Here's how the part is built. I have some questions about the finished solid (model axes, mm). A direction names the side the tool comes from. Round coordinates to 2 decimals unless told otherwise and drop trailing zeros. Order: outer loops, then holes, each group sorted by start corner. A loop starts at its lowest first (then second) coordinate and runs counter-clockwise, first axis right, second up. Notation, with made-up numbers: M -7.75,13 L 8.25,13 A9 cw 8.25,20 Z; hole C 27.25,4.25 d6. An arc over 180 degrees is marked long. Answer as CSV lines item,"result". Start each with the question number.
```python
from build123d import *

# Parameters (mm, degrees)
F1_DEPTH  = 6.096
F2_R      = 4.7625
F3_DEPTH  = 140.971
F4_R      = 3.175
F5_DEPTH  = 117.476
F6_R      = 2.0193
F6_R_2    = 1.6002
F7_DEPTH  = 12.7
F8_R      = 1.6002
F8_R_2    = 2.0193
F9_DEPTH  = 10.16
F10_R     = 1.6002
F10_R_2   = 2.0193
F11_DEPTH = 10.16


with BuildPart() as f1:
    # F0 (on Front) → F1 (new body, symmetric)
    with BuildSketch(Plane.XZ):
        with BuildLine():
            Line((-70.485, 0), (0, 0))
            Line((0, 0), (70.485, 0))
            Line((70.485, 0), (70.485, 117.475))
            Line((70.485, 117.475), (57.785, 117.475))
            Line((57.785, 117.475), (57.785, 45.3136))
            ThreePointArc((57.785, 45.3136), (57.4966846366, 43.4219130898), (56.6579198847, 41.7020064627))
            Line((56.6579198847, 41.7020064627), (38.4969198847, 15.4384064627))
            ThreePointArc((38.4969198847, 15.4384064627), (36.2226336699, 13.426117046), (33.274, 12.7))
            Line((33.274, 12.7), (0, 12.7))
            Line((0, 12.7), (-33.274, 12.7))
            ThreePointArc((-33.274, 12.7), (-36.2226336699, 13.426117046), (-38.4969198847, 15.4384064627))
            Line((-38.4969198847, 15.4384064627), (-56.6579198847, 41.7020064627))
            ThreePointArc((-56.6579198847, 41.7020064627), (-57.4966846366, 43.4219130898), (-57.785, 45.3136))
            Line((-57.785, 45.3136), (-57.785, 117.475))
            Line((-57.785, 117.475), (-70.485, 117.475))
            Line((-70.485, 117.475), (-70.485, 0))
        make_face()
    extrude(amount=F1_DEPTH, both=True)

    # F2 (on face) → F3 (cut, through all)
    with BuildSketch(Plane.YZ.offset(70.485)):
        with Locations((0, 111.125)):
            Circle(F2_R)
        with Locations((0, 85.725)):
            Circle(F2_R)
    extrude(amount=-F3_DEPTH, mode=Mode.SUBTRACT)

    # F4 (on face) → F5 (cut, through all)
    with BuildSketch(Plane(origin=(0, 0, 0), x_dir=(1, 0, 0), z_dir=(0, 0, -1))):
        with Locations((-22.225, 0)):
            Circle(F4_R)
        with Locations((22.225, 0)):
            Circle(F4_R)
    extrude(amount=-F5_DEPTH, mode=Mode.SUBTRACT)

    # F6 (on face) → F7 (cut)
    with BuildSketch(Plane(origin=(0, 0, 0), x_dir=(1, 0, 0), z_dir=(0, 0, -1))):
        with Locations((-50.8, 0)):
            Circle(F6_R)
        with Locations((-58.293, 0)):
            Circle(F6_R_2)
        with Locations((50.8, 0)):
            Circle(F6_R)
        with Locations((58.293, 0)):
            Circle(F6_R_2)
    extrude(amount=-F7_DEPTH, mode=Mode.SUBTRACT)

    # F8 (on face) → F9 (cut)
    with BuildSketch(Plane.YZ.offset(70.485)):
        with Locations((0, 6.35)):
            Circle(F8_R)
        with Locations((0, 47.625)):
            Circle(F8_R)
        with Locations((0, 15.875)):
            Circle(F8_R_2)
    extrude(amount=-F9_DEPTH, mode=Mode.SUBTRACT)

    # F10 (on face) → F11 (cut)
    with BuildSketch(Plane(origin=(-70.485, 0, 0), x_dir=(0, -1, 0), z_dir=(-1, 0, 0))):
        with Locations((0, 6.35)):
            Circle(F10_R)
        with Locations((0, 15.875)):
            Circle(F10_R_2)
        with Locations((0, 47.625)):
            Circle(F10_R)
    extrude(amount=-F11_DEPTH, mode=Mode.SUBTRACT)


solid = f1.part
```
Item 1: If we section it at D-D on y = 0: Count the separate pieces of the cut face and the enclosed holes in it, and give its area (3 significant figures).
Item 2: If we section it at A-A on z = 92: Please give me the cut outline in (x, y) (3 decimals), and give its area (3 significant figures).
Item 3: Which directions (+Z, -Z, +X, -X, +Y, -Y) give clear straight access to the entire face, cutting with the end or side of a thin tool? Please do faces 4 (the cylindrical face through (-65.476, 0.438, 13.904)), 5 (the flat face through (0, 0, 12.7)), 6 (the cylindrical face through (65.48, -0.35, 4.79)).
Item 4: If we section it at B-B on z = 6.35: Please give me the cut outline in (x, y) (3 decimals), and give its area (3 significant figures).
Item 5: For P1, Ø1.9, axis at y = 0, z = 47.625, coming from the +X side (3 decimals); P2, Ø4, axis at x = 58.293, y = 0, coming from the -Z side; P3, Ø3, axis at x = 45.5, y = 2.5, coming from the +Z side; P4, Ø1.6, axis at y = 0, z = 6.5, coming from the -X side (3 decimals), each with a flat end and sliding along its axis, tell me the tip position at first contact or that it passes through.
Item 6: If I drill on line 1 along Z through (x, y) = (67.25, 0) (1 decimal); line 2 along Z through (x, y) = (-59.5, 0.25) (3 decimals); line 3 along X through (y, z) = (5, 105) (3 decimals), over which ranges is the centre line in solid material (lowest first)?
Item 7: If we section it at C-C on x = -22.5: Please give me the cut outline in (y, z).
Item 8: We'd pull the mould along Y, two halves only. Please class faces 1 (the flat face through (47.7, -0.09, 28.75)), 2 (the flat face through (-6, -6.096, 11)), 3 (the cylindrical face through (-65.48, 0.35, 4.79)): pulls with the +Y half, pulls with the -Y half, needs draft (parallel to the pull), parting line crosses it, or undercut.
Geometry says:
1,separate pieces,"7"
1,enclosed holes,"0"
1,area,"4,060 mm²"
2,outline,"M -70.485,-6.096 L -57.785,-6.096 L -57.785,6.096 L -70.485,6.096 Z; M 57.785,-6.096 L 70.485,-6.096 L 70.485,6.096 L 57.785,6.096 Z"
2,area,"310 mm²"
3,face 4,"-X"
3,face 5,"+Z, +Y, -Y"
3,face 6,"+X"
4,outline,"M -70.485,-6.096 L 70.485,-6.096 L 70.485,-1.6 L 60.325,-1.6 L 60.325,1.6 L 70.485,1.6 L 70.485,6.096 L -70.485,6.096 L -70.485,1.6 L -60.325,1.6 L -60.325,-1.6 L -70.485,-1.6 Z; hole C -58.293,0 d3.2; hole C -50.8,0 d4.039; hole C -22.225,0 d6.35; hole C 22.225,0 d6.35; hole C 50.8,0 d4.039; hole C 58.293,0 d3.2"
4,area,"1,550 mm²"
5,P1,"x = 60.325"
5,P2,"z = 0"
5,P3,"z = 27.74"
5,P4,"x = -60.325"
6,line 1,"0 to 4.7, 8 to 13.9, 17.9 to 46, 49.2 to 81, 90.5 to 106.4, 115.9 to 117.5"
6,line 2,"12.7 to 80.969, 90.481 to 106.369, 115.881 to 117.475"
6,line 3,"-70.485 to -57.785, 57.785 to 70.485"
7,outline,"M -6.1,0 L -3.16,0 L -3.16,12.7 L -6.1,12.7 Z; M 3.16,0 L 6.1,0 L 6.1,12.7 L 3.16,12.7 Z"
8,face 1,"needs draft"
8,face 2,"pulls with the -Y half"
8,face 3,"undercut"
